Could you check a few things on this model? Use its own coordinates, in mm. Face numbers are marked on the shaded views. A direction names the side the tool comes from. Coordinates: 2 decimals unless noted, no trailing zeros. Order: outer loops, then holes, each group sorted by start corner. A loop starts at its lowest first (then second) coordinate and runs counter-clockwise, first axis right, second up. Notation, with made-up numbers: (-24, -24) - (35, -24) arc R29 ccw to (35, -4) - close; hole circle Ø4 at (46.5, -39). An arc over 180 degrees is marked (long way). One line per item, written item: value.
from build123d import *

# Parameters (mm, degrees)
BOSS_EXTRUDE1_DEPTH = 15
SKETCH2_W           = 25
SKETCH2_H           = 13.5
CUT_EXTRUDE1_DEPTH  = 3
SKETCH3_W           = 25
SKETCH3_H           = 13.5
CUT_EXTRUDE2_DEPTH  = 3
BOSS_EXTRUDE2_DEPTH = 5
BOSS_EXTRUDE3_DEPTH = 5
SKETCH6_R           = 3.25
CUT_EXTRUDE3_DEPTH  = 8.5
SKETCH7_R           = 2.125
CUT_EXTRUDE4_DEPTH  = 5
SKETCH8_R           = 3.65
CUT_EXTRUDE5_DEPTH  = 2.5
CHAMFER3_SIZE       = 0.5
FILLET1_R           = 3
SKETCH9_R           = 4.5
SKETCH9_R_2         = 3.85
BOSS_EXTRUDE4_DEPTH = 1.8
CHAMFER4_SIZE       = 5
CHAMFER5_SIZE       = 1
CHAMFER6_SIZE       = 0.5


with BuildPart() as part:
    # Sketch1 → Boss-Extrude1 (new body)
    with BuildSketch(Plane.XY):
        Polygon((0, 0), (20, 0), (20, 10), (35, 10), (35, 0), (55, 0), (55, 5), (40, 5), (40, 18.5), (15, 18.5), (15, 5), (0, 5), align=None)
    extrude(amount=BOSS_EXTRUDE1_DEPTH)

    # Sketch2 → Cut-Extrude1 (cut)
    with BuildSketch(Plane.XY.offset(15)):
        with Locations((27.5, 11.75)):
            Rectangle(SKETCH2_W, SKETCH2_H)
    extrude(amount=-CUT_EXTRUDE1_DEPTH, mode=Mode.SUBTRACT)

    # Sketch3 → Cut-Extrude2 (cut)
    with BuildSketch(Plane(origin=(0, 0, 0), x_dir=(-1, 0, 0), z_dir=(0, 0, -1))):
        with Locations((-27.5, 11.75)):
            Rectangle(SKETCH3_W, SKETCH3_H)
    extrude(amount=-CUT_EXTRUDE2_DEPTH, mode=Mode.SUBTRACT)

    # Sketch4 → Boss-Extrude2 (add)
    with BuildSketch(Plane(origin=(20, 0, 0), x_dir=(0, 0, -1), z_dir=(1, 0, 0))):
        Polygon((-12, 18.5), (-15, 5), (-12, 5), align=None)
        Polygon((-3, 5), (0, 5), (-3, 18.5), align=None)
    extrude(amount=-BOSS_EXTRUDE2_DEPTH)

    # Sketch5 → Boss-Extrude3 (add)
    with BuildSketch(Plane.ZY.offset(-35)):
        Polygon((0, 5), (3, 18.5), (3, 5), align=None)
        Polygon((12, 18.5), (12, 5), (15, 5), align=None)
    extrude(amount=-BOSS_EXTRUDE3_DEPTH)

    # Sketch6 → Cut-Extrude3 (cut)
    with BuildSketch(Plane(origin=(0, 18.5, 0), x_dir=(1, 0, 0), z_dir=(0, 1, 0))):
        with Locations((27.5, -7.5)):
            Circle(SKETCH6_R)
    extrude(amount=-CUT_EXTRUDE3_DEPTH, mode=Mode.SUBTRACT)

    # Sketch7 → Cut-Extrude4 (cut)
    with BuildSketch(Plane(origin=(0, 5, 0), x_dir=(1, 0, 0), z_dir=(0, 1, 0))):
        with Locations((7.5, -7.5)):
            Circle(SKETCH7_R)
        with Locations((47.5, -7.5)):
            Circle(SKETCH7_R)
    extrude(amount=-CUT_EXTRUDE4_DEPTH, mode=Mode.SUBTRACT)

    # Sketch8 → Cut-Extrude5 (cut)
    with BuildSketch(Plane(origin=(0, 5, 0), x_dir=(1, 0, 0), z_dir=(0, 1, 0))):
        with Locations((7.5, -7.5)):
            Circle(SKETCH8_R)
        with Locations((47.5, -7.5)):
            Circle(SKETCH8_R)
    extrude(amount=-CUT_EXTRUDE5_DEPTH, mode=Mode.SUBTRACT)

    # Chamfer3
    chamfer3_edges = [part.edges().sort_by_distance(p)[0] for p in [
        (3.85, 5, 7.5),
        (43.85, 5, 7.5),
    ]]
    chamfer(chamfer3_edges, length=CHAMFER3_SIZE)

    # Fillet1
    fillet1_edges = [part.edges().sort_by_distance(p)[0] for p in [
        (55, 2.5, 0),
        (0, 2.5, 0),
        (55, 2.5, 15),
        (0, 2.5, 15),
    ]]
    fillet(fillet1_edges, radius=FILLET1_R)

    # Sketch9 → Boss-Extrude4 (add)
    with BuildSketch(Plane(origin=(0, 18.5, 0), x_dir=(1, 0, 0), z_dir=(0, 1, 0))):
        with Locations((27.5, -7.5)):
            Circle(SKETCH9_R)
        with Locations((27.5, -7.5)):
            Circle(SKETCH9_R_2, mode=Mode.SUBTRACT)
    extrude(amount=BOSS_EXTRUDE4_DEPTH)

    # Chamfer4
    chamfer4_edges = [part.edges().sort_by_distance(p)[0] for p in [
        (40, 18.5, 7.5),
        (15, 18.5, 7.5),
    ]]
    chamfer(chamfer4_edges, length=CHAMFER4_SIZE)

    # Chamfer5
    chamfer5_edges = [part.edges().sort_by_distance(p)[0] for p in [
        (0, 5, 7.5),
        (0.878679656, 5, 14.121320344),
        (0.878679656, 5, 0.878679656),
        (55, 5, 7.5),
        (46, 5, 15),
        (46, 5, 0),
        (54.121320344, 5, 14.121320344),
        (54.121320344, 5, 0.878679656),
        (27.5, 10, 12),
        (27.5, 10, 3),
        (9, 5, 15),
        (9, 5, 0),
    ]]
    chamfer(chamfer5_edges, length=CHAMFER5_SIZE)

    # Chamfer6
    chamfer6_edges = [part.edges().sort_by_distance(p)[0] for p in [
        (23, 20.3, 7.5),
    ]]
    chamfer(chamfer6_edges, length=CHAMFER6_SIZE)


solid = part.part
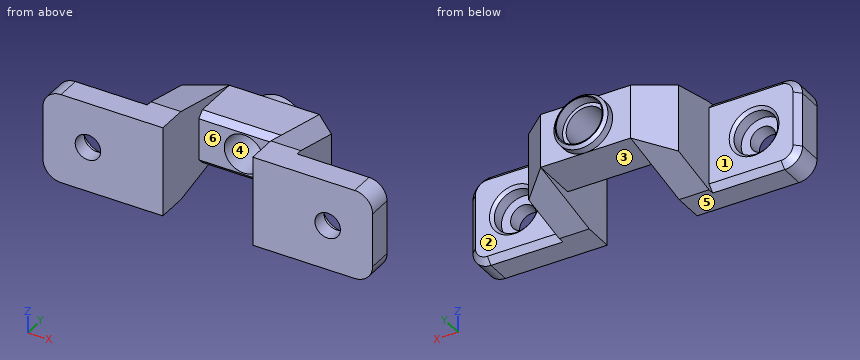
Item 1: I want a section at A-A on y = 3.25. Please give me the cut outline in (x, z), then the cut area to 3 significant figures.
Conclusion:
outline: (0, 3) arc R3 ccw to (3, 0) - (20, 0) - (20, 15) - (3, 15) arc R3 ccw to (0, 12) - close; (35, 0) - (52, 0) arc R3 ccw to (55, 3) - (55, 12) arc R3 ccw to (52, 15) - (35, 15) - close; hole circle Ø7.3 at (7.5, 7.5); hole circle Ø7.3 at (47.5, 7.5)
area: 509 mm²
Item 2: I want a section at B-B on x = 7.5. Please give me the cut outline in (y, z) (3 decimals), then the cut area to 3 significant figures.
Conclusion:
outline: (0, 0) - (4, 0) - (5, 1) - (5, 3.35) - (4.5, 3.85) - (2.5, 3.85) - (2.5, 5.375) - (0, 5.375) - close; (0, 9.625) - (2.5, 9.625) - (2.5, 11.15) - (4.5, 11.15) - (5, 11.65) - (5, 14) - (4, 15) - (0, 15) - close
area: 44.9 mm²
Item 3: I want a section at C-C on z = 7.5. Give the number of separate pieces and of enclosed holes in the cut face, then the cut area to 3 significant figures.
Conclusion:
separate pieces: 4
enclosed holes: 0
area: 325 mm²
Item 4: If I drill on probe 1 along X at (y, z) = (3.45, 7.5); probe 2 along X at (y, z) = (19.15, 7.5); probe 3 along X at (y, z) = (1, 3), over which ranges is the centre line in solid material (lowest first)?
Conclusion:
probe 1: 0 to 3.85, 11.15 to 20, 35 to 43.85, 51.15 to 55
probe 2: 23 to 23.65, 31.35 to 32
probe 3: 0 to 20, 35 to 55
Item 5: For the marked faces 1, 2 and 3, which set-ups out of +Z, -Z, +X, -X, +Y, -Y let a thin tool reach every point of the face, with its end or its side?
Conclusion:
face 1: +Z, -Z, -X, +Y
face 2: +Z, -Z, +X, +Y
face 3: -Z, +Y, -Y
Item 6: I'm going to push flat-ended pins straight in: pin 1 Ø4 at (x, z) = (48, 9.5) entering from +Y; pin 2 Ø7.5 at (y, z) = (8, 10.5) entering from +X; pin 3 Ø10 at (x, y) = (43, 12) entering from -Z; pin 4 Ø6 at (x, z) = (27.5, 7.5) entering from -Y. Where does each tip first touch, or does it pass through?
Conclusion:
pin 1: y = 4.91
pin 2: x = 54.75
pin 3: z = 0.67
pin 4: through
Item 7: Thinking about a two-plate mould opening in Z: for the marked faces 4, 5 and 6, which applies, pulls with the +Z half, pulls with the -Z half, needs draft (parallel to the pull), parting line crosses it, or undercut?
Conclusion:
face 4: undercut
face 5: pulls with the -Z half
face 6: needs draft
Item 8: I want a section at D-D on y = 6.5. Please give me the cut outline in (x, z).
Conclusion:
outline: (15, 0.33) - (20, 0.33) - (20, 14.67) - (15, 14.67) - close; (35, 0.33) - (40, 0.33) - (40, 14.67) - (35, 14.67) - close
